from build123d import *

# Parameters (mm, degrees)
F3_DEPTH = 40.001
F2_W     = 2.5
F2_H     = 8
F4_DEPTH = 8
F5_R     = 2.25
F6_DEPTH = 25
F7_SIZE  = 0.99999
F8_SIZE  = 0.5


# Not quite as in the source:
# - a fillet or chamfer is up to 0.001 mm smaller than in the source, because OpenCascade refuses the exact size


with BuildPart() as f1:
    # F0 (on Front) → F1 (revolve)
    with BuildSketch(Plane.XZ):
        Polygon((-6.85, 0), (0, 0), (0, 40), (-10, 40), (-10, 30), (-6.85, 30), align=None)
    revolve(axis=Axis((0, 0, 20), (0, 0, -1)))

    # F2 (on face) → F3 (cut, through all)
    with BuildSketch(Plane.XY.offset(40)):
        Polygon((4.25, -2.4537386441), (4.25, 2.4537386441), (0, 4.9074772881), (-4.25, 2.4537386441), (-4.25, -2.4537386441), (0, -4.9074772881), align=None)
    extrude(amount=-F3_DEPTH, mode=Mode.SUBTRACT)

    # F2 (on face) → F4 (cut)
    with BuildSketch(Plane.XY.offset(40)):
        with Locations((-6.5, 0)):
            Rectangle(F2_W, F2_H)
        with Locations((6.5, 0)):
            Rectangle(F2_W, F2_H)
    extrude(amount=-F4_DEPTH, mode=Mode.SUBTRACT)

    # F5 (on face) → F6 (cut, symmetric)
    with BuildSketch(Plane(origin=(-5.25, 0, 0), x_dir=(0, -1, 0), z_dir=(-1, 0, 0))):
        with Locations((0, 35.5)):
            Circle(F5_R)
    extrude(amount=F6_DEPTH, both=True, mode=Mode.SUBTRACT)

    # F7 (size 1 in the source; OpenCascade refuses exactly that, so slightly less here)
    f7_edges = [f1.edges().sort_by_distance(p)[0] for p in [
        (10, 0, 40),
        (10, 0, 30),
        (-2.125, 3.680608, 40),
        (2.125, 3.680608, 40),
        (4.25, 0, 40),
        (2.125, -3.680608, 40),
        (-2.125, -3.680608, 40),
        (-4.25, 0, 40),
    ]]
    chamfer(f7_edges, length=F7_SIZE)

    # F8
    f8_edges = [f1.edges().sort_by_distance(p)[0] for p in [
        (6.85, 0, 0),
        (4.25, 0, 0),
        (2.125, -3.680608, 0),
        (-2.125, -3.680608, 0),
        (-4.25, 0, 0),
        (-2.125, 3.680608, 0),
        (2.125, 3.680608, 0),
    ]]
    chamfer(f8_edges, length=F8_SIZE)


solid = f1.part
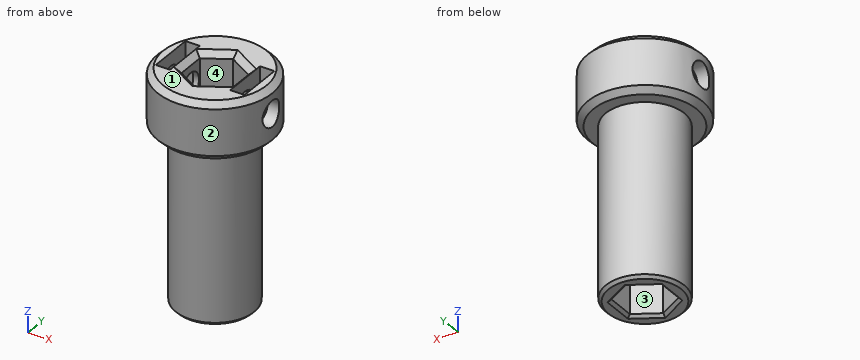
The model under review builds one solid part; all positions refer to its coordinate system, in mm. Face numbers are marked on the shaded views. Round coordinates to 2 decimals unless told otherwise and drop trailing zeros. Loops run counter-clockwise (first coordinate to the right, second up) from the corner with the lowest first, then second, coordinate; pieces in that order, holes last. Notation, with made-up numbers: (-29, -26) -> (6, -26) arc R15 ccw to (6, -5) -> close; hole circle Ø4 at (54.5, 55). An arc over 180 degrees is marked (long way). One line per question, with ' | ' between items. Start each with the question number.
Item 1: Add section A-A, the plane z = 3. Write out the cut boundary in (x, y), then the cut area to 3 significant figures.
Item 2: Add section B-B, the plane y = 0. Count the separate pieces of the cut face and the enclosed holes in it, then the cut area to 3 significant figures.
Item 3: Wall thickness on line 1 along X through (y, z) = (-2.5, 25); line 2 along Z through (x, y) = (-4.25, 6.5); line 3 along Z through (x, y) = (8.25, -1): over which ranges is each line inside the solid? List them lowest first. Write a range as [from, to].
Item 4: Draft analysis for pull direction X (two halves, no side actions). For the marked faces 1, 2, 3 and 4, state which applies: +X half, -X half, draft (parallel to the pull), parting line (faces both ways), or undercut.
Item 5: For pin 1 (5.5 mm diameter, centred on y = -0.5, z = 20.5, fed in from +X); pin 2 (5.5 mm diameter, centred on y = 0, z = 10.5, fed in from -X); pin 3 (4 mm diameter, centred on x = -5, z = 33.5, fed in from +Y); pin 4 (4 mm diameter, centred on y = 0, z = 35.5, fed in from -X), all flat-tipped, find the tip position at first contact; note any pin that passes through.
Item 6: Add section D-D, the plane z = 30.5. Write out the cut boundary in (x, y), then the cut area to 3 significant figures.
Return value:
1) outline: circle Ø13.7 at (0, 0); hole (-4.25, -2.45) -> (0, -4.91) -> (4.25, -2.45) -> (4.25, 2.45) -> (0, 4.91) -> (-4.25, 2.45) -> close | area: 84.8 mm2
2) separate pieces: 6 | enclosed holes: 0 | area: 198 mm2
3) line 1: x = [-6.38, -4.17], [4.17, 6.38] | line 2: z = [30, 40] | line 3: z = [30, 33.48], [37.52, 40]
4) face 1: draft | face 2: parting line | face 3: undercut | face 4: undercut
5) pin 1: stops at x = 6.85 | pin 2: stops at x = -6.85 | pin 3: stops at y = 9.54 | pin 4: passes through
6) outline: circle Ø19 at (0, 0); hole (-4.25, -2.45) -> (0, -4.91) -> (4.25, -2.45) -> (4.25, 2.45) -> (0, 4.91) -> (-4.25, 2.45) -> close | area: 221 mm2
